```python
from build123d import *

# Parameters (mm, degrees)
F0_R     = 3.390494
F0_R_2   = 12.7
F1_DEPTH = 6.35


with BuildPart() as f1:
    # F0 (on Front) → F1 (new body)
    with BuildSketch(Plane.XZ):
        Polygon((-80.893202, 16.455771), (-76.127474, 3.323797), (-82.521767, 2.158814), (-75.548098, -9.946096), (-81.64295, -12.203737), (-72.673232, -22.913782), (-78.283453, -26.195485), (-67.590225, -35.185244), (-72.545354, -39.391296), (-60.453525, -46.387621), (-64.603, -51.390222), (-51.479974, -56.180533), (-54.697717, -61.827682), (-40.94223, -64.266428), (-43.130471, -70.386539), (-29.160478, -70.39962), (-30.252728, -76.806738), (-16.492699, -74.393756), (-16.455771, -80.893202), (-3.323797, -76.127474), (-2.158814, -82.521767), (9.946096, -75.548098), (12.203737, -81.64295), (22.913782, -72.673232), (26.195485, -78.283453), (35.185244, -67.590225), (39.391296, -72.545354), (46.387621, -60.453525), (51.390222, -64.603), (56.180533, -51.479974), (61.827682, -54.697717), (64.266428, -40.94223), (70.386539, -43.130471), (70.39962, -29.160478), (76.806738, -30.252728), (74.393756, -16.492699), (80.893202, -16.455771), (76.127474, -3.323797), (82.521767, -2.158814), (75.548098, 9.946096), (81.64295, 12.203737), (72.673232, 22.913782), (78.283453, 26.195485), (67.590225, 35.185244), (72.545354, 39.391296), (60.453525, 46.387621), (64.603, 51.390222), (51.479974, 56.180533), (54.697717, 61.827682), (40.94223, 64.266428), (43.130471, 70.386539), (29.160478, 70.39962), (30.252728, 76.806738), (16.492699, 74.393756), (16.455771, 80.893202), (3.323797, 76.127474), (2.158814, 82.521767), (-9.946096, 75.548098), (-12.203737, 81.64295), (-22.913782, 72.673232), (-26.195485, 78.283453), (-35.185244, 67.590225), (-39.391296, 72.545354), (-46.387621, 60.453525), (-51.390222, 64.603), (-56.180533, 51.479974), (-61.827682, 54.697717), (-64.266428, 40.94223), (-70.386539, 43.130471), (-70.39962, 29.160478), (-76.806738, 30.252728), (-74.393756, 16.492699), align=None)
        with BuildLine():
            ThreePointArc((-11.128394, -12.738895), (-6.579044, -19.606941), (-6.170858, -27.834944))
            Line((-6.170858, -27.834944), (-11.222449, -50.621197))
            ThreePointArc((-11.222449, -50.621197), (-20.055193, -61.459456), (-34.023103, -60.840828))
            ThreePointArc((-34.023103, -60.840828), (-49.290236, -49.291485), (-60.839966, -34.024645))
            ThreePointArc((-60.839966, -34.024645), (-61.458908, -20.055655), (-50.619858, -11.222152))
            Line((-50.619858, -11.222152), (-27.834944, -6.170858))
            ThreePointArc((-27.834944, -6.170858), (-19.606941, -6.579044), (-12.738895, -11.128394))
            Line((-12.738895, -11.128394), (-11.128394, -12.738895))
        make_face(mode=Mode.SUBTRACT)
        with Locations((0, -66.426293)):
            Circle(F0_R, mode=Mode.SUBTRACT)
        with Locations((0, -53.726293)):
            Circle(F0_R, mode=Mode.SUBTRACT)
        with Locations((0, -41.026293)):
            Circle(F0_R, mode=Mode.SUBTRACT)
        with Locations((0, -28.326293)):
            Circle(F0_R, mode=Mode.SUBTRACT)
        with BuildLine():
            ThreePointArc((12.738895, -11.128394), (19.606941, -6.579044), (27.834944, -6.170858))
            Line((27.834944, -6.170858), (50.621197, -11.222449))
            ThreePointArc((50.621197, -11.222449), (61.459456, -20.055193), (60.840828, -34.023103))
            ThreePointArc((60.840828, -34.023103), (49.291485, -49.290236), (34.024645, -60.839966))
            ThreePointArc((34.024645, -60.839966), (20.055655, -61.458908), (11.222152, -50.619858))
            Line((11.222152, -50.619858), (6.170858, -27.834944))
            ThreePointArc((6.170858, -27.834944), (6.579044, -19.606941), (11.128394, -12.738895))
            Line((11.128394, -12.738895), (12.738895, -11.128394))
        make_face(mode=Mode.SUBTRACT)
        with Locations((-66.426293, 0)):
            Circle(F0_R, mode=Mode.SUBTRACT)
        with Locations((-53.726293, 0)):
            Circle(F0_R, mode=Mode.SUBTRACT)
        with Locations((-41.026293, 0)):
            Circle(F0_R, mode=Mode.SUBTRACT)
        with Locations((-28.326293, 0)):
            Circle(F0_R, mode=Mode.SUBTRACT)
        with BuildLine():
            ThreePointArc((-12.738895, 11.128394), (-19.606941, 6.579044), (-27.834944, 6.170858))
            Line((-27.834944, 6.170858), (-50.621197, 11.222449))
            ThreePointArc((-50.621197, 11.222449), (-61.459456, 20.055193), (-60.840828, 34.023103))
            ThreePointArc((-60.840828, 34.023103), (-49.291485, 49.290236), (-34.024645, 60.839966))
            ThreePointArc((-34.024645, 60.839966), (-20.055655, 61.458908), (-11.222152, 50.619858))
            Line((-11.222152, 50.619858), (-6.170858, 27.834944))
            ThreePointArc((-6.170858, 27.834944), (-6.579044, 19.606941), (-11.128394, 12.738895))
            Line((-11.128394, 12.738895), (-12.738895, 11.128394))
        make_face(mode=Mode.SUBTRACT)
        Circle(F0_R_2, mode=Mode.SUBTRACT)
        with Locations((28.326293, 0)):
            Circle(F0_R, mode=Mode.SUBTRACT)
        with Locations((41.026293, 0)):
            Circle(F0_R, mode=Mode.SUBTRACT)
        with Locations((0, 28.326293)):
            Circle(F0_R, mode=Mode.SUBTRACT)
        with Locations((0, 41.026293)):
            Circle(F0_R, mode=Mode.SUBTRACT)
        with BuildLine():
            Line((50.619858, 11.222152), (27.834944, 6.170858))
            ThreePointArc((27.834944, 6.170858), (19.606941, 6.579044), (12.738895, 11.128394))
            ThreePointArc((12.738895, 11.128394), (11.960782, 11.960782), (11.128394, 12.738895))
            ThreePointArc((11.128394, 12.738895), (6.579044, 19.606941), (6.170858, 27.834944))
            Line((6.170858, 27.834944), (11.222449, 50.621197))
            ThreePointArc((11.222449, 50.621197), (20.055193, 61.459456), (34.023103, 60.840828))
            ThreePointArc((34.023103, 60.840828), (49.290236, 49.291485), (60.839966, 34.024645))
            ThreePointArc((60.839966, 34.024645), (61.458908, 20.055655), (50.619858, 11.222152))
        make_face(mode=Mode.SUBTRACT)
        with Locations((53.726293, 0)):
            Circle(F0_R, mode=Mode.SUBTRACT)
        with Locations((66.426293, 0)):
            Circle(F0_R, mode=Mode.SUBTRACT)
        with Locations((0, 53.726293)):
            Circle(F0_R, mode=Mode.SUBTRACT)
        with Locations((0, 66.426293)):
            Circle(F0_R, mode=Mode.SUBTRACT)
    extrude(amount=F1_DEPTH)


solid = f1.part
```
The model under review builds one solid part; all positions refer to its coordinate system, in mm. A direction names the side the tool comes from. Round coordinates to 2 decimals unless told otherwise and drop trailing zeros. Answer as a JSON object with one key per item and string values.
(1) Tool access review of faces 4 (the flat face through (79.28, -3.13, -2.75)), 5 (the flat face through (-8.732, -3.131, 39.387)), 6 (the flat face through (2.75, -3.13, 79.28)): name each direction out of +Z, -Z, +X, -X, +Y, -Y from which nothing blocks a thin tool from reaching the whole face with its end or side.
Resolved:
{"face 4": "+X, +Y, -Y", "face 5": "+Y, -Y", "face 6": "+Z, +Y, -Y"}
(2) Clearance check with flat-ended pins moving along their axes: P1, Ø6, axis at x = -53.73, z = 0, coming from the +Y side; P2, Ø1, axis at y = -5.5, z = 59.5, coming from the +X side; P3, Ø1, axis at x = -20.5, y = -1, coming from the -Z side. State where each tip first meets the part, or that it passes through.
Resolved:
{"P1": "through", "P2": "x = 53.66", "P3": "z = -75.18"}
(3) To check wall thickness, follow line 1 along X through (y, z) = (-2, -40.5); line 2 along X through (y, z) = (-1.25, -38); line 3 along Z through (x, y) = (-69, -4). State the ranges of each line that lie inside material, in increasing order.
Resolved:
{"line 1": "-70.63 to -56.74, -8.98 to -3.35, 3.35 to 8.98, 56.74 to 70.39", "line 2": "-70.91 to -58.44, -8.42 to -1.53, 1.53 to 8.42, 58.44 to 70.39", "line 3": "-41.44 to -36.38, -34 to -2.21, 2.21 to 42.63"}
(4) Take a section at A-A on x = 0. Count the separate pieces of the cut face and the enclosed holes in it, and give its area (3 significant figures).
Resolved:
{"separate pieces": "10", "enclosed holes": "0", "area": "526 mm²"}
(5) Draft analysis for pull direction Z (two halves, no side actions). For faces 1 (the cylindrical face through (-0.441, -3.131, -63.065)), 2 (the flat face through (-23.469, -3.131, -75.617)), 3 (the flat face through (-37.259, -3.131, 70.033)), state which applies: released by +Z, released by -Z, zero draft, split by the parting line, or undercut.
Resolved:
{"face 1": "undercut", "face 2": "released by -Z", "face 3": "released by +Z"}
